Print and shaded views of the part. All mm, measured from the part's lowest x, y and z. Coordinates: 2 decimals unless noted, no trailing zeros. Loops run counter-clockwise (first coordinate to the right, second up) from the corner with the lowest first, then second, coordinate; pieces in that order, holes last. Notation, with made-up numbers: M 28,37 L 47,37 A21 cw 47,61 Z; hole C 40.5,88 d8. An arc over 180 degrees is marked long. Use a Markdown table: item, result. Add a question column.
1) Band-saw the part on C-C (z = 37.5). List the corners of the cut face in (x, y).
2) Wall check: probe 1 along Y at (x, z) = (2, 82.5); probe 2 along Z at (x, y) = (6.25, 231.5); probe 3 along Z at (x, y) = (1.75, 323.5). Give the ranges that are in metal, low to high. Write a range as from..to.
3) Band-saw the part on B-B (y = 313.5). List the corners of the cut face in (x, z).
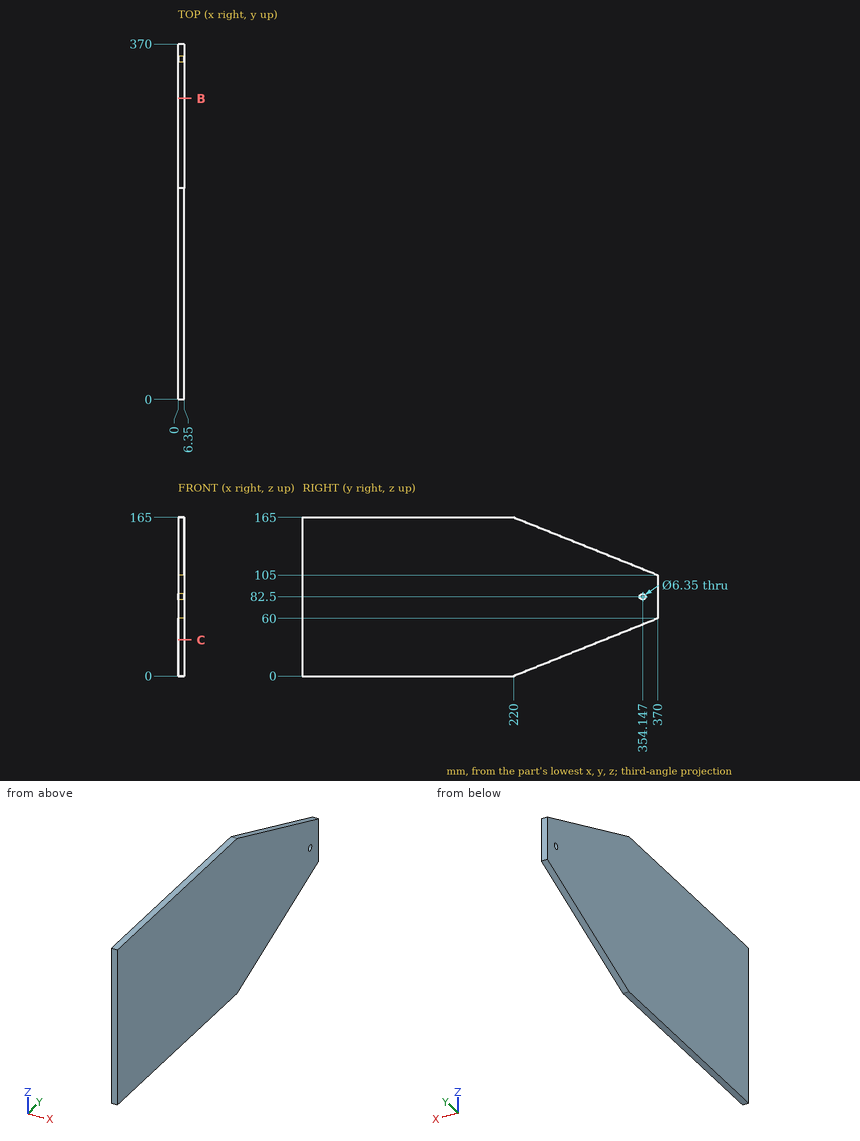
Entries:
| question | item | result |
|---|---|---|
| 1 | outline | M 0,0 L 6.35,0 L 6.35,313.75 L 0,313.75 Z |
| 2 | probe 1 | 0..350.97, 357.32..370 |
| 2 | probe 2 | 4.6..160.4 |
| 2 | probe 3 | 41.4..123.6 |
| 3 | outline | M 0,37.4 L 6.35,37.4 L 6.35,127.6 L 0,127.6 Z |
